Input: part model. Units: mm. Frame: model coordinates. A direction names the side the tool comes from. Coordinates: 2 decimals unless noted, no trailing zeros. Write each loop counter-clockwise with the first axis right and the second up, starting at its lowest first coordinate (ties: lowest second). Pieces come first, ordered by that corner, then holes. Notation, with made-up numbers: (47.5, -35) - (69.5, -35) arc R31 cw to (69.5, -8) - close; hole circle Ø3 at (62, -5.75). An arc over 180 degrees is marked (long way). Use a Markdown table: item, result. Add a question column.
Q1. Set-up query: faces 4 (the face through (0.381, 0, 9)), 5 (the face through (5.944, 3, 12)). Return all of +Z, -Z, +X, -X, +Y, -Y with unobstructed straight access to the full face (end or side cutting, diameter ignored); none if empty.
Q2. Pin query (flat end, axial travel): P1, Ø1, axis at y = 2, z = 7, coming from the +X side; P2, Ø6.5, axis at x = 11.13, y = 0, coming from the +Z side; P3, Ø6, axis at x = 9.5, z = 11, coming from the -Y side; P4, Ø4.5, axis at y = 0, z = 12.7, coming from the -X side. Return the tip coordinate at first contact, or that it passes through.
Q3. Mould query, pull axis Y, two halves, no side actions, for faces 1 (the face through (3, 0, 18.237)), 2 (the face through (5, -6.35, 7)), 3 (the face through (3.132, -0.089, 10.683)). Classes: released by +Y, released by -Y, zero draft, split by the parting line, or undercut.
Q4. Material intervals for probe 1 along X at (y, z) = (0, 2.85); probe 2 along Z at (x, y) = (3.1, 0); probe 3 along X at (y, z) = (-4.5, 11), sorted ascending. Write a range as from..to.
Q5. Section query A-A (z = 12.7). Return the cut outline in (x, y).
Q6. Section query B-B (y = 0). Return the cut outline in (x, z), then the cut area to 3 significant figures.
Q7. Section query C-C (x = 3). Return the cut outline in (y, z), then the cut area to 3 significant figures.
Q8. Section query D-D (z = 7.25). Return the cut outline in (x, y).
from build123d import *

# Parameters (mm, degrees)
EXTRUDE1_DEPTH = 6.35
FILLET1_R      = 0.508


with BuildPart() as part:
    # Sketch1 → Extrude1 (new, symmetric)
    with BuildSketch(Plane(origin=(0, 0, 0), x_dir=(1, 0, 0), z_dir=(0, 1, 0))):
        Polygon((5.9436, -18.2372), (5.9436, -5.5626), (16.256, -5.5626), (16.256, 0), (0.381, 0), (0.381, -18.2372), align=None)
    extrude(amount=EXTRUDE1_DEPTH, both=True)

    # Sketch2 → #10-32 Tapped Hole2 (revolve, cut)
    with BuildSketch(Plane(origin=(0.381, 0, 12.7), x_dir=(0, 0, 1), z_dir=(0, 1, 0))):
        Polygon((0, 0), (0, 5.5626), (2.667, 5.5626), (2.0193, 4.9149), (2.0193, 0.6477), (2.667, 0), align=None)
    revolve(axis=Axis((-5.969, 0, 12.7), (1, 0, 0)), mode=Mode.SUBTRACT)

    # Sketch4 → #10-32 Tapped Hole1 (revolve, cut)
    with BuildSketch(Plane.YZ.offset(11.1252)):
        Polygon((0, 0), (0, 5.5626), (2.667, 5.5626), (2.0193, 4.9149), (2.0193, 0.6477), (2.667, 0), align=None)
    revolve(axis=Axis((11.1252, 0, -6.35), (0, 0, 1)), mode=Mode.SUBTRACT)

    # Fillet1
    fillet1_edges = [part.edges().sort_by_distance(p)[0] for p in [
        (5.9436, 6.35, 11.8999),
        (16.256, 6.35, 2.7813),
        (0.381, 6.35, 9.1186),
        (16.256, -6.35, 2.7813),
        (5.9436, -6.35, 11.8999),
        (0.381, -6.35, 9.1186),
    ]]
    fillet(fillet1_edges, radius=FILLET1_R)


solid = part.part
Values follow:
| question | item | result |
|---|---|---|
| 1 | face 4 | +Z, -Z, -X, +Y, -Y |
| 1 | face 5 | +Z, +X, +Y, -Y |
| 2 | P1 | x = 5.94 |
| 2 | P2 | z = 5.56 |
| 2 | P3 | through |
| 2 | P4 | x = 0.8 |
| 3 | face 1 | zero draft |
| 3 | face 2 | released by -Y |
| 3 | face 3 | undercut |
| 4 | probe 1 | 0.38..9.11, 13.14..16.26 |
| 4 | probe 2 | 0..10.68, 14.72..18.24 |
| 4 | probe 3 | 0.38..5.94 |
| 5 | outline | (0.38, -5.84) arc R0.51 ccw to (0.89, -6.35) - (5.44, -6.35) arc R0.51 ccw to (5.94, -5.84) - (5.94, -2.67) - (5.3, -2.02) - (1.03, -2.02) - (0.38, -2.67) - close; (0.38, 2.67) - (1.03, 2.02) - (5.3, 2.02) - (5.94, 2.67) - (5.94, 5.84) arc R0.51 ccw to (5.44, 6.35) - (0.89, 6.35) arc R0.51 ccw to (0.38, 5.84) - close |
| 6 | outline | (0.38, 0) - (8.46, 0) - (9.11, 0.65) - (9.11, 4.91) - (8.46, 5.56) - (5.94, 5.56) - (5.94, 10.03) - (5.3, 10.68) - (1.03, 10.68) - (0.38, 10.03) - close; (0.38, 15.37) - (1.03, 14.72) - (5.3, 14.72) - (5.94, 15.37) - (5.94, 18.24) - (0.38, 18.24) - close; (13.14, 0.65) - (13.79, 0) - (16.26, 0) - (16.26, 5.56) - (13.79, 5.56) - (13.14, 4.91) - close |
| 6 | area | 112 mm2 |
| 7 | outline | (-6.35, 0) - (6.35, 0) - (6.35, 18.24) - (-6.35, 18.24) - close; hole circle Ø4.04 at (0, 12.7) |
| 7 | area | 219 mm2 |
| 8 | outline | (0.38, -5.84) arc R0.51 ccw to (0.89, -6.35) - (5.44, -6.35) arc R0.51 ccw to (5.94, -5.84) - (5.94, 5.84) arc R0.51 ccw to (5.44, 6.35) - (0.89, 6.35) arc R0.51 ccw to (0.38, 5.84) - close |
